from build123d import *

# Parameters (mm, degrees)
SKETCH1_R           = 12.5
BOSS_EXTRUDE1_DEPTH = 107
SKETCH2_R           = 12.4
BOSS_EXTRUDE2_DEPTH = 85
SKETCH3_R           = 10
BOSS_EXTRUDE3_DEPTH = 10


with BuildPart() as part:
    # Sketch1 → Boss-Extrude1 (new body)
    with BuildSketch(Plane(origin=(0, 0, 0), x_dir=(1, 0, 0), z_dir=(0, 1, 0))):
        Circle(SKETCH1_R)
    extrude(amount=BOSS_EXTRUDE1_DEPTH)

    # Sketch2 → Boss-Extrude2 (add)
    with BuildSketch(Plane(origin=(0, 107, 0), x_dir=(1, 0, 0), z_dir=(0, 1, 0))):
        Circle(SKETCH2_R)
    extrude(amount=BOSS_EXTRUDE2_DEPTH)

    # Sketch3 → Boss-Extrude3 (add)
    with BuildSketch(Plane.XZ):
        Circle(SKETCH3_R)
    extrude(amount=BOSS_EXTRUDE3_DEPTH)


solid = part.part
For this review, take the finished solid that the model builds, in its own axes (mm). A direction names the side the tool comes from. Give positions to 0.01 mm unless a question says otherwise; leave off trailing zeros. Loops run counter-clockwise (first coordinate to the right, second up) from the corner with the lowest first, then second, coordinate; pieces in that order, holes last. Notation, with made-up numbers: M 65,55.25 L 85,55.25 A30 ccw 85,93.25 Z; hole C 54.25,26 d3. An arc over 180 degrees is marked long. Answer as a JSON object with one key per item and string values. Group by question number.
Q1. Add section A-A on x = -0.75. Give the boundary of the cut face in (y, z), and give its area (3 significant figures).
Q2. Insertion check: P1, Ø12, axis at y = 165.5, z = 2, coming from the +X side; P2, Ø5, axis at x = 4.5, y = 60, coming from the +Z side; P3, Ø3, axis at y = 11.5, z = -4, coming from the +X side; P4, Ø10, axis at x = -8, z = -7.5, coming from the -Y side. Each pin has a flat end and moves straight along its axis. Give the tip position at first contact, or say it passes through.
Q3. Add section D-D on y = 18. Give the boundary of the cut face in (x, z).
Q4. Add section B-B on z = -6.75. Give the boundary of the cut face in (x, y).
Q5. For probe 1 along Y at (x, z) = (-9.25, -4.75); probe 2 along Z at (x, y) = (1, 66); probe 3 along X at (y, z) = (174.5, -0.75), list the stretches that pass through material, from the lowest coordinate up. Write a range as [from, to].
Q6. Add section C-C on y = 155. Give the boundary of the cut face in (x, z).
Q7. Tool access review of faces 1 (the flat face through (0, 192, 0)), 2 (the flat face through (-0.1, 0, -10.2)): name each direction out of +Z, -Z, +X, -X, +Y, -Y from which nothing blocks a thin tool from reaching the whole face with its end or side.
Checked values:
{
 "1": {"outline": "M -10,-9.97 L 0,-9.97 L 0,-12.48 L 107,-12.48 L 107,-12.38 L 192,-12.38 L 192,12.38 L 107,12.38 L 107,12.48 L 0,12.48 L 0,9.97 L -10,9.97 Z", "area": "4,970 mm²"},
 "2": {"P1": "x = 12.4", "P2": "z = 12.34", "P3": "x = 12.25", "P4": "y = -10"},
 "3": {"outline": "C 0,0 d25"},
 "4": {"outline": "M -10.52,0 L -7.38,0 L -7.38,-10 L 7.38,-10 L 7.38,0 L 10.52,0 L 10.52,107 L 10.4,107 L 10.4,192 L -10.4,192 L -10.4,107 L -10.52,107 Z"},
 "5": {"probe 1": "[0, 192]", "probe 2": "[-12.46, 12.46]", "probe 3": "[-12.38, 12.38]"},
 "6": {"outline": "C 0,0 d24.8"},
 "7": {"face 1": "+Z, -Z, +X, -X, +Y", "face 2": "-Y"}
}
